Autodesk Inventor part; units mm, degrees
ref_plane "Work Plane1" through (0, 0, 0) normal (1, 0, 0) x (0, 0, -1)
ref_plane "YZ Plane" through (0, 0, 0) normal (1, 0, 0) x (0, 1, 0)
ref_plane "XZ Plane" through (0, 0, 0) normal (0, 1, 0) x (-1, 0, 0)
sketch "Sketch1" plane through (0, 0, 0) normal (1, 0, 0) x (0, 1, 0)
  line L0 (9.8672, 30.93) -> (-65.8248, 30.93)
  line L1 (-65.8248, 30.93) -> (-65.8248, 21.786)
  line L2 (-65.8248, 21.786) -> (9.8672, 21.786)
  line L3 (9.8672, 21.786) -> (9.8672, 30.93)
  circle A0 centre (-65.8248, 26.358) radius 4.572
  circle A1 centre (-65.8248, 26.358) radius 6.8324
  point P0 (0, 0)
  dimension "d0" = 75.692
  dimension "d1" = 9.144
extrude "Extrusion3" add sketch "Sketch1" along normal mid plane 4.064 contours L3 L2 A1 L0 | A1 L2 A0 L0 | A0 L1 picked at (-59.8517, 25.4679) picked at (-64.4517, 25.6968)
extrude "Extrusion4" add sketch "Sketch1" along normal mid plane 12.192 contours A1 L2 A0 L0 | L0 A0 L2 A1
extrude "Extrusion5" cut sketch "Sketch1" along normal mid plane 12.192 contours A0 L1 | L1 A0
ref_plane "Work Plane1" through (0, 0, 0) normal (1, 0, 0) x (0, 0, -1)
sketch "Sketch2" plane through (0, 0, 0) normal (1, 0, 0) x (0, 0, -1)
  line L0 (-30.93, 9.8672) -> (-21.786, 9.8672)
  line L1 (-26.358, 9.8672) -> (-26.358, 27.0122)
  circle A0 centre (-26.358, 27.0122) radius 18.034
  point P0 (0, 0)
  dimension "d12" = 17.145
  dimension "d13" = 36.068
extrude "Extrusion6" add sketch "Sketch2" along normal mid plane 12.192
fillet "Fillet1" radius 3.175 2 edges at (2.032, 8.9782, 26.358) (-2.032, 8.9782, 26.358)
properties part number "pendulum"
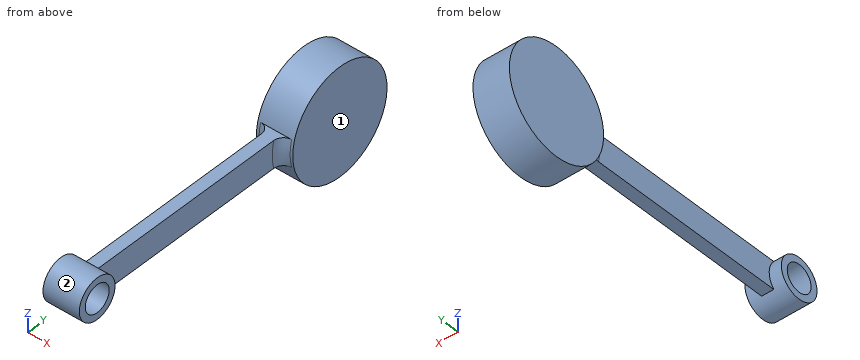
For this review, take the finished solid that the model builds, in its own axes (mm). Face numbers are marked on the shaded views. Round coordinates to 2 decimals unless told otherwise and drop trailing zeros. Write each loop counter-clockwise with the first axis right and the second up, starting at its lowest first coordinate (ties: lowest second). Pieces come first, ordered by that corner, then holes. Notation, with made-up numbers: (54.5, 29) - (64.5, 29) arc R18 ccw to (64.5, 58) - close; hole circle Ø1 at (-6, 6.25). An arc over 180 degrees is marked (long way). Write item = value, one per line. Start each with the question number.
1. Consider section B-B on y = -12. State the section outline as (x, z) points, plus the area to 3 significant figures.
2. Wall thickness on L1, parallel to Y at x = -4.75, z = 26.5 (3 decimals); L2, parallel to Z at x = 0.5, y = -9.5; L3, parallel to Z at x = 1.25, y = -62: over which ranges is each line inside the solid? List them lowest first.
3. Consider section D-D on x = -3.75. State the section outline as (y, z) points.
4. For pin 1 Ø1 at (x, z) = (3.5, 17) entering from -Y; pin 2 Ø1.5 at (x, z) = (-0.5, 39) entering from +Y; pin 3 Ø1 at (x, y) = (-0.5, -36) entering from +Z; pin 4 Ø6 at (y, z) = (-10, 18.5) entering from -X, all flat-tipped, find the tip position at first contact; note any pin that passes through.
5. Consider section A-A on x = 3.25. State the section outline as (y, z) points.
6. Draft analysis for pull direction Y (two halves, no side actions). For the marked faces 1 and 2, state which applies: released by +Y, released by -Y, zero draft, split by the parting line, or undercut.
7. Consider section C-C on z = 14. State the section outline as (x, y) points, plus the area to 3 significant figures.
Evaluation:
q1.outline = (-2.03, 21.79) - (2.03, 21.79) - (2.03, 30.93) - (-2.03, 30.93) - close
q1.area = 37.2 mm2
q2.L1 = -72.656 to -70.395, -61.255 to -58.994, 8.946 to 45.046
q2.L2 = 21.79 to 30.93
q2.L3 = 20.7 to 23.85, 28.86 to 32.02
q3.outline = circle Ø13.66 at (-65.82, 26.36); (9.2, 21.79) - (9.57, 21.79) arc R18.03 ccw (long way) to (9.57, 30.93) - (9.2, 30.93) arc R18.39 ccw to start; hole circle Ø9.14 at (-65.82, 26.36)
q4.pin_1 = 11.3
q4.pin_2 = 40.57
q4.pin_3 = 30.93
q4.pin_4 = through
q5.outline = circle Ø13.66 at (-65.82, 26.36); (8.87, 21.79) - (9.57, 21.79) arc R18.03 ccw (long way) to (9.57, 30.93) - (8.87, 30.93) arc R18.71 ccw to start; hole circle Ø9.14 at (-65.82, 26.36)
q6.face_1 = zero draft
q6.face_2 = undercut
q7.outline = (-6.1, 13.88) - (6.1, 13.88) - (6.1, 40.15) - (-6.1, 40.15) - close
q7.area = 320 mm2
